```python
from build123d import *

# Parameters (mm, degrees)
SKETCH_1_R      = 4
EXTRUDE_1_DEPTH = 1


with BuildPart() as part:
    # 草图1 → 凸台-拉伸1 (new body)
    with BuildSketch(Plane(origin=(0, 0, 0), x_dir=(1, 0, 0), z_dir=(0, 1, 0))):
        with BuildLine():
            Line((-44, -56), (44, -56))
            ThreePointArc((44, -56), (58.142135624, -50.142135624), (64, -36))
            Line((64, -36), (64, 36))
            ThreePointArc((64, 36), (58.142135624, 50.142135624), (44, 56))
            Line((44, 56), (-44, 56))
            ThreePointArc((-44, 56), (-58.142135624, 50.142135624), (-64, 36))
            Line((-64, 36), (-64, -36))
            ThreePointArc((-64, -36), (-58.142135624, -50.142135624), (-44, -56))
        make_face()
        with Locations(Location((-28, 45, 0), (0, 0, 270))):
            Circle(SKETCH_1_R, mode=Mode.SUBTRACT)
        with Locations(Location((0, 45, 0), (0, 0, 270))):
            Circle(SKETCH_1_R, mode=Mode.SUBTRACT)
        with Locations(Location((28, 45, 0), (0, 0, 90))):
            Circle(SKETCH_1_R, mode=Mode.SUBTRACT)
        with Locations(Location((-53, 31.5, 0), (0, 0, 270))):
            Circle(SKETCH_1_R, mode=Mode.SUBTRACT)
        with Locations(Location((-53, 0, 0), (0, 0, 270))):
            Circle(SKETCH_1_R, mode=Mode.SUBTRACT)
        with Locations(Location((-53, -31.5, 0), (0, 0, 90))):
            Circle(SKETCH_1_R, mode=Mode.SUBTRACT)
        with Locations(Location((53, 31.5, 0), (0, 0, 90))):
            Circle(SKETCH_1_R, mode=Mode.SUBTRACT)
        with Locations(Location((53, 0, 0), (0, 0, 90))):
            Circle(SKETCH_1_R, mode=Mode.SUBTRACT)
        with Locations(Location((53, -31.5, 0), (0, 0, 270))):
            Circle(SKETCH_1_R, mode=Mode.SUBTRACT)
        with Locations(Location((28, -45, 0), (0, 0, 270))):
            Circle(SKETCH_1_R, mode=Mode.SUBTRACT)
        with Locations(Location((0, -45, 0), (0, 0, 90))):
            Circle(SKETCH_1_R, mode=Mode.SUBTRACT)
        with Locations(Location((-28, -45, 0), (0, 0, 90))):
            Circle(SKETCH_1_R, mode=Mode.SUBTRACT)
        with BuildLine():
            Line((-39, -28), (39, -28))
            ThreePointArc((39, -28), (43.242640687, -26.242640687), (45, -22))
            Line((45, -22), (45, 22))
            ThreePointArc((45, 22), (43.242640687, 26.242640687), (39, 28))
            Line((39, 28), (-39, 28))
            ThreePointArc((-39, 28), (-43.242640687, 26.242640687), (-45, 22))
            Line((-45, 22), (-45, -22))
            ThreePointArc((-45, -22), (-43.242640687, -26.242640687), (-39, -28))
        make_face(mode=Mode.SUBTRACT)
    extrude(amount=EXTRUDE_1_DEPTH)


solid = part.part
```
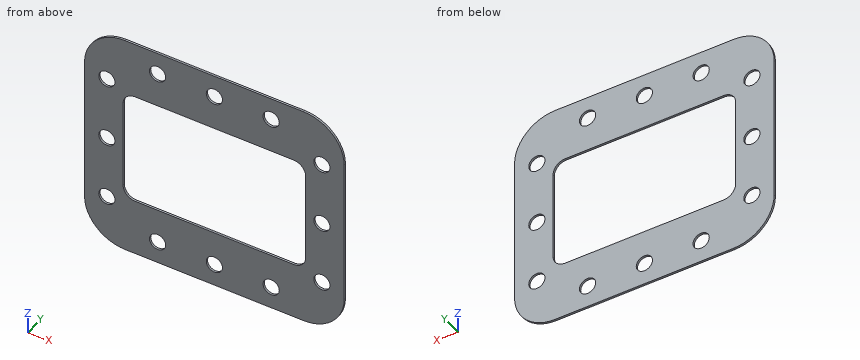
Geometry check sheet. Reference: the model listing, model coordinates, mm. Round coordinates to 2 decimals unless told otherwise and drop trailing zeros. Order: outer loops, then holes, each group sorted by start corner. A loop starts at its lowest first (then second) coordinate and runs counter-clockwise, first axis right, second up. Notation, with made-up numbers: (59.25, 33.25) - (78.25, 33.25) arc R19 cw to (78.25, 37.25) - close; hole circle Ø5 at (-23.5, 73). An arc over 180 degrees is marked (long way). Use a Markdown table: item, result. Add a question column.
(1) Sectioned sample at C-C, the plane z = -31.5. Enter the section's corners in (x, y), and give its area (3 significant figures).
(2) Sectioned sample at A-A, the plane z = 0. Enter the section's corners in (x, y), and give its area (3 significant figures).
(3) Material ranges on line 1 along X through (y, z) = (0.55, -31.5); line 2 along X through (y, z) = (0.65, 41.5); line 3 along X through (y, z) = (0.35, -3), recorded low to high. Write a range as [from, to].
(4) Sectioned sample at D-D, the plane x = 14.5. Enter the section's corners in (y, z), and give its area (3 significant figures).
(5) Sectioned sample at B-B, the plane x = 0. Enter the section's corners in (y, z), and give its area (3 significant figures).
Answers below:
| question | item | result |
|---|---|---|
| 1 | outline | (-64, 0) - (-57, 0) - (-57, 1) - (-64, 1) - close; (-49, 0) - (49, 0) - (49, 1) - (-49, 1) - close; (57, 0) - (64, 0) - (64, 1) - (57, 1) - close |
| 1 | area | 112 mm² |
| 2 | outline | (-64, 0) - (-57, 0) - (-57, 1) - (-64, 1) - close; (-49, 0) - (-45, 0) - (-45, 1) - (-49, 1) - close; (45, 0) - (49, 0) - (49, 1) - (45, 1) - close; (57, 0) - (64, 0) - (64, 1) - (57, 1) - close |
| 2 | area | 22.0 mm² |
| 3 | line 1 | [-64, -57], [-49, 49], [57, 64] |
| 3 | line 2 | [-63.23, -29.94], [-26.06, -1.94], [1.94, 26.06], [29.94, 63.23] |
| 3 | line 3 | [-64, -55.65], [-50.35, -45], [45, 50.35], [55.65, 64] |
| 4 | outline | (0, -56) - (1, -56) - (1, -28) - (0, -28) - close; (0, 28) - (1, 28) - (1, 56) - (0, 56) - close |
| 4 | area | 56.0 mm² |
| 5 | outline | (0, -56) - (1, -56) - (1, -49) - (0, -49) - close; (0, -41) - (1, -41) - (1, -28) - (0, -28) - close; (0, 28) - (1, 28) - (1, 41) - (0, 41) - close; (0, 49) - (1, 49) - (1, 56) - (0, 56) - close |
| 5 | area | 40.0 mm² |
